Input: part model. Units: mm. Frame: model coordinates. Give positions to 0.01 mm unless a question says otherwise; leave off trailing zeros. Loops run counter-clockwise (first coordinate to the right, second up) from the corner with the lowest first, then second, coordinate; pieces in that order, holes last. Notation, with made-up numbers: M -4.5,65.25 L -0.5,65.25 A19 ccw -0.5,80.25 Z; hole C -28.5,34 d6. An arc over 180 degrees is marked long. Answer as a JSON object with one key per item and string values. Group by question number.
1) First-contact query: P1, Ø2, axis at x = 0, z = -539.6, coming from the -Y side. Flat tip, straight axial feed; report the tip coordinate or a pass-through.
2) Ray query, L1, parallel to X at y = -1.25, z = -599.6 (3 decimals); L2, parallel to Z at x = -1.5, y = 0.5; L3, parallel to Z at x = -1, y = -3. Return the intervals inside material, ascending.
3) Section query B-B on z = -539.6. Return loops of the section in (x, y) (3 decimals), plus the area to 3 significant figures.
4) Section query A-A on x = 0. Return loops of the section in (y, z) (3 decimals), plus the area to 3 significant figures.
5) Section query C-C on y = 0.5. Return loops of the section in (x, z) (3 decimals).
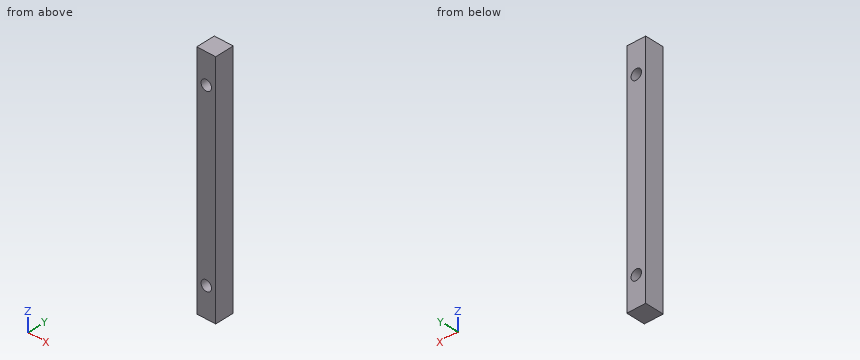
from build123d import *

# Parameters (mm, degrees)
BOSS_EXTRUDE1_DEPTH      = 609.6
BOSS_EXTRUDE1_DEPTH_BACK = 609.6
SKETCH3_W                = 6.35
SKETCH3_H                = 6.35
SKETCH4_W                = 7.35
SKETCH4_H                = 7.35
CUT_EXTRUDE1_DEPTH       = 1140.208848829
SKETCH5_R                = 1.75
CUT_EXTRUDE2_DEPTH       = 610.641339744


with BuildPart() as part:
    # Sketch3 → Boss-Extrude1 (new, two sides: drawn at the far end of the back side and taken through both)
    with BuildSketch(Plane.XY.offset(-BOSS_EXTRUDE1_DEPTH_BACK)):
        Rectangle(SKETCH3_W, SKETCH3_H)
    extrude(amount=BOSS_EXTRUDE1_DEPTH + BOSS_EXTRUDE1_DEPTH_BACK)

    # Sketch4 → Cut-Extrude1 (cut, through all)
    with BuildSketch(Plane(origin=(0, 0, -529.6), x_dir=(-1, 0, 0), z_dir=(0, 0, -1))):
        Rectangle(SKETCH4_W, SKETCH4_H)
    extrude(amount=-CUT_EXTRUDE1_DEPTH, mode=Mode.SUBTRACT)

    # Sketch5 → Cut-Extrude2 (cut, through all)
    with BuildSketch(Plane(origin=(0, 3.175, 0), x_dir=(1, 0, 0), z_dir=(0, 1, 0))):
        with Locations(Location((0, 599.6, 0), (0, 0, 270))):
            Circle(SKETCH5_R)
        with Locations(Location((0, 539.6, 0), (0, 0, 270))):
            Circle(SKETCH5_R)
    extrude(amount=-CUT_EXTRUDE2_DEPTH, mode=Mode.SUBTRACT)


solid = part.part
Output:
{
 "1": {"P1": "passes through"},
 "2": {"L1": "x = -3.175 to -1.75, 1.75 to 3.175", "L2": "z = -609.6 to -600.5, -598.7 to -540.5, -538.7 to -529.6", "L3": "z = -609.6 to -601.04, -598.16 to -541.04, -538.16 to -529.6"},
 "3": {"outline": "M -3.175,-3.175 L -1.75,-3.175 L -1.75,3.175 L -3.175,3.175 Z; M 1.75,-3.175 L 3.175,-3.175 L 3.175,3.175 L 1.75,3.175 Z", "area": "18.1 mm^2"},
 "4": {"outline": "M -3.175,-609.6 L 3.175,-609.6 L 3.175,-601.35 L -3.175,-601.35 Z; M -3.175,-597.85 L 3.175,-597.85 L 3.175,-541.35 L -3.175,-541.35 Z; M -3.175,-537.85 L 3.175,-537.85 L 3.175,-529.6 L -3.175,-529.6 Z", "area": "464 mm^2"},
 "5": {"outline": "M -3.175,-609.6 L 3.175,-609.6 L 3.175,-529.6 L -3.175,-529.6 Z; hole C 0,-599.6 d3.5; hole C 0,-539.6 d3.5"}
}
